```python
from build123d import *

# Parameters (mm, degrees)
SKETCH3_R          = 3
CUT_EXTRUDE1_DEPTH = 13.97
FILLET1_R          = 3


with BuildPart() as part:
    # Sketch2 → Revolve1 (revolve)
    with BuildSketch(Plane(origin=(0, 0, 0), x_dir=(0, 0, -1), z_dir=(1, 0, 0))):
        with BuildLine():
            Line((0, 0), (0, 15.5067))
            ThreePointArc((0, 15.5067), (3.928862053, 13.879312053), (5.55625, 9.95045))
            Line((5.55625, 9.95045), (5.55625, 4.7625))
            Line((5.55625, 4.7625), (3.96875, 4.7625))
            Line((3.96875, 4.7625), (3.96875, 0))
            Line((3.96875, 0), (0, 0))
        make_face()
    revolve(axis=Axis((0, 0, 0), (0, 1, 0)))

    # Sketch3 → Cut-Extrude1 (cut)
    with BuildSketch(Plane.XZ):
        Circle(SKETCH3_R)
    extrude(amount=-CUT_EXTRUDE1_DEPTH, mode=Mode.SUBTRACT)

    # Fillet1
    fillet1_edges = [part.edges().sort_by_distance(p)[0] for p in [
        (-3, 13.97, 0),
    ]]
    fillet(fillet1_edges, radius=FILLET1_R)


solid = part.part
```
Read the model definition and answer for the solid it produces. Units are mm, in the model's axes. A direction names the side the tool comes from. Give positions to 0.01 mm unless a question says otherwise; leave off trailing zeros. Order: outer loops, then holes, each group sorted by start corner. A loop starts at its lowest first (then second) coordinate and runs counter-clockwise, first axis right, second up. Notation, with made-up numbers: (89.25, 16) -> (118.25, 16) arc R24 cw to (118.25, 53) -> close; hole circle Ø1 at (70.5, 67.5). An arc over 180 degrees is marked (long way). Write item = value, one per line.
1. A cutting plane is placed at C-C, the plane z = 0. Write down the section's boundary in (x, y), and give its area (3 significant figures).
Numbers:
outline = (-5.56, 4.76) -> (-3.97, 4.76) -> (-3.97, 0) -> (-3, 0) -> (-3, 10.97) arc R3 cw to (3, 10.97) -> (3, 0) -> (3.97, 0) -> (3.97, 4.76) -> (5.56, 4.76) -> (5.56, 9.95) arc R5.56 ccw to (-5.56, 9.95) -> close
area = 64.0 mm²
2. A cutting plane is placed at A-A, the plane y = 4.5. Write down the section's boundary in (x, z), and give its area (3 significant figures).
Numbers:
outline = circle Ø7.94 at (0, 0); hole circle Ø6 at (0, 0)
area = 21.2 mm²
3. A cutting plane is placed at D-D, the plane x = 2.5. Write down the section's boundary in (y, z).
Numbers:
outline = (0, -3.08) -> (4.76, -3.08) -> (4.76, -4.96) -> (9.95, -4.96) arc R4.96 ccw to (9.95, 4.96) -> (4.76, 4.96) -> (4.76, 3.08) -> (0, 3.08) -> (0, 1.66) -> (10.97, 1.66) arc R1.66 cw to (10.97, -1.66) -> (0, -1.66) -> close
4. Straight lines are drawn through the part: line 1 along Z through (x, y) = (0, 5); line 2 along Z through (x, y) = (0, 3.5); line 3 along X through (y, z) = (5.75, 1.75). For each, find the intervals that lie inside material, in ascending order.
Numbers:
line_1 = -5.56 to -3, 3 to 5.56
line_2 = -3.97 to -3, 3 to 3.97
line_3 = -5.27 to -2.44, 2.44 to 5.27
5. For faces 4 (the face through (-1, 4.762, 4)), 5 (the face through (-1.67, 7.32, -5.3)), determine the directions among +Z, -Z, +X, -X, +Y, -Y from which every point of the face is accessible in a straight line to the end or side of a thin tool.
Numbers:
face_4 = -Y
face_5 = +Y, -Y
6. Given pin 1 (2 mm diameter, centred on x = 4, z = 3, fed in from -Y); pin 2 (5 mm diameter, centred on y = 8, z = 3.5, fed in from +X); pin 3 (2 mm diameter, centred on x = 3.5, y = 3.5, fed in from -Z), each flat-ended and moving along its own axis, determine where each tip first touches the part or whether it passes through.
Numbers:
pin_1 = 4.76
pin_2 = 5.47
pin_3 = -3.08
7. The mould has two halves that part along X. Classify faces 1 (the face through (3.874, 2.348, 0.86)), 2 (the face through (-3, 0, -1)), 3 (the face through (-3, 5, 0)): +X half, -X half, draft (parallel to the pull), parting line (faces both ways), or undercut.
Numbers:
face_1 = parting line
face_2 = draft
face_3 = undercut
8. A cutting plane is placed at B-B, the plane x = 0. Write down the section's boundary in (y, z).
Numbers:
outline = (0, -3.97) -> (4.76, -3.97) -> (4.76, -5.56) -> (9.95, -5.56) arc R5.56 ccw to (9.95, 5.56) -> (4.76, 5.56) -> (4.76, 3.97) -> (0, 3.97) -> (0, 3) -> (10.97, 3) arc R3 cw to (10.97, -3) -> (0, -3) -> close
